```python
from build123d import *

# Parameters (mm, degrees)
F0_W      = 1000
F0_H      = 5.5340008238
F0_H_2    = 212.9319983523
F1_DEPTH  = 25
F2_W      = 900
F2_H      = 124
F3_DEPTH  = 15
F4_W      = 976
F4_H      = 200
F5_DEPTH  = 380
F6_T      = -12
F7_W      = 380
F7_H      = 45
F8_DEPTH  = 5
F9_W      = 380
F9_H      = 45
F10_DEPTH = 5
F11_R     = 4
F12_DEPTH = 12


# Not quite as in the source:
# - a shell that OpenCascade refuses in one call is made with other operations: the cavity is built on its own and cut out


with BuildPart() as f1:
    # F0 (on Front) → F1 (new body)
    with BuildSketch(Plane.XZ):
        with Locations((0, 109.2329995881)):
            Rectangle(F0_W, F0_H)
        Rectangle(F0_W, F0_H_2)
        with Locations((0, -109.2329995881)):
            Rectangle(F0_W, F0_H)
    extrude(amount=F1_DEPTH)

    # F2 (on face) → F3 (cut)
    with BuildSketch(Plane.XZ.offset(25)):
        Rectangle(F2_W, F2_H)
    extrude(amount=-F3_DEPTH, mode=Mode.SUBTRACT)

    # F4 (on face) → F5 (join)
    with BuildSketch(Plane(origin=(0, 0, 0), x_dir=(-1, 0, 0), z_dir=(0, 1, 0))):
        Rectangle(F4_W, F4_H)
    extrude(amount=F5_DEPTH)

    # F6: a shell. OpenCascade refuses it in one call, so the cavity is built on its own and cut out:
    # the body offset inwards by the wall thickness, plus a prism from it out through each open face.
    f6_core = offset(f1.part, amount=F6_T, kind=Kind.INTERSECTION, mode=Mode.PRIVATE)
    f6_exits = [f6_core.faces().sort_by_distance(p)[0] for p in [
        (0, 178, 88),
    ]]
    add(f6_core, mode=Mode.SUBTRACT)
    extrude(f6_exits, amount=-F6_T, mode=Mode.SUBTRACT)

    # F7 (on face) → F8 (join)
    with BuildSketch(Plane(origin=(-488, 0, 0), x_dir=(0, -1, 0), z_dir=(-1, 0, 0))):
        with Locations((-190, 0)):
            Rectangle(F7_W, F7_H)
    extrude(amount=F8_DEPTH)

    # F9 (on face) → F10 (join)
    with BuildSketch(Plane.YZ.offset(488)):
        with Locations((190, 0)):
            Rectangle(F9_W, F9_H)
    extrude(amount=F10_DEPTH)

    # F11 (on face) → F12 (cut, through all)
    with BuildSketch(Plane.XZ.offset(10)):
        with Locations((-55, 0)):
            Circle(F11_R)
        with BuildLine():
            ThreePointArc((59, 0), (55, 4), (51, 0))
            ThreePointArc((51, 0), (55, -4), (59, 0))
        make_face()
    extrude(amount=-F12_DEPTH, mode=Mode.SUBTRACT)


solid = f1.part
```
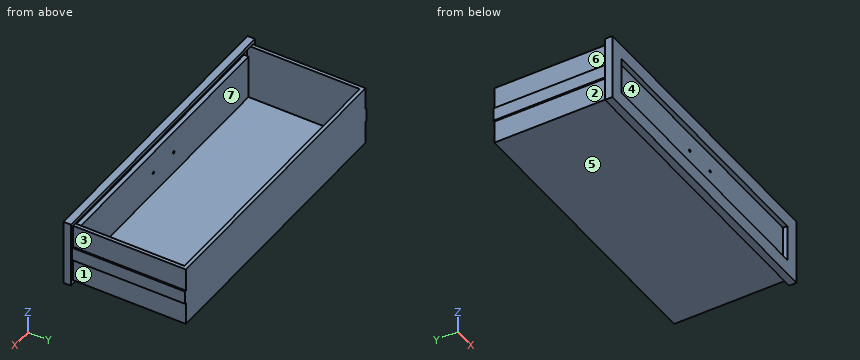
Build history of the part. All positions in model axes, mm. Face numbers are marked on the shaded views. A direction names the side the tool comes from. Give positions to 0.01 mm unless a question says otherwise; leave off trailing zeros. Order: outer loops, then holes, each group sorted by start corner. A loop starts at its lowest first (then second) coordinate and runs counter-clockwise, first axis right, second up. Notation, with made-up numbers: M 34,34 L 73,34 A15 ccw 73,47 Z; hole C 37.25,15.5 d4. An arc over 180 degrees is marked long. Return JSON: item names as keys, results as strings.
Q1. Band-saw the part on C-C (x = 178.5). Give the cut face in (y, z).
Answer list:
{"outline": "M -25,-112 L 0,-112 L 0,-100 L 380,-100 L 380,100 L 368,100 L 368,-88 L -12,-88 L -12,-100 L -13,-100 L -13,-74 L 2,-74 L 2,74 L -13,74 L -13,100 L 0,100 L 0,112 L -25,112 L -25,62 L -10,62 L -10,-62 L -25,-62 Z"}
Q2. 3-axis set-ups, long thin cutter, end or side, ignore diameter. For the marked faces 1, 2, 3 and 4: which of +Z, -Z, +X, -X, +Y, -Y reach the whole face in a straight line?
Answer list:
{"face 1": "-Z, +X, +Y", "face 2": "-Z, -X, +Y", "face 3": "+Z, +X, +Y", "face 4": "-Y"}
Q3. Flat gauge pins, fed straight in: pin 1 (2 mm diameter, centred on x = -4, y = 129, fed in from +Z); pin 2 (10 mm diameter, centred on y = 283, z = 61, fed in from -X); pin 3 (5 mm diameter, centred on y = 191.5, z = 17.5, fed in from -X). Where does each tip first touch, or does it go through?
Answer list:
{"pin 1": "stops at z = -88", "pin 2": "stops at x = -488", "pin 3": "stops at x = -493"}
Q4. Wall check: probe 1 along Z at (x, y) = (-55, -6); probe 2 along X at (y, z) = (-5.5, 52.5); probe 3 along X at (y, z) = (334.5, -53). Give the ranges that are in metal, low to high. Write a range as from..to.
Answer list:
{"probe 1": "z = -112..-88, -74..-4, 4..74, 100..112", "probe 2": "x = -500..-476, -462..462, 476..500", "probe 3": "x = -488..-476, 476..488"}
Q5. Two-plate mould, pull along X, no slides. Class the marked faces 5, 6 and 7: pulls with the +X half, pulls with the -X half, needs draft (parallel to the pull), parting line crosses it, or undercut.
Answer list:
{"face 5": "needs draft", "face 6": "pulls with the -X half", "face 7": "undercut"}
Q6. Band-saw the part on B-B (y = 35). Give the cut face in (x, z).
Answer list:
{"outline": "M -493,-22.5 L -488,-22.5 L -488,-100 L 488,-100 L 488,-22.5 L 493,-22.5 L 493,22.5 L 488,22.5 L 488,100 L 476,100 L 476,-88 L -476,-88 L -476,100 L -488,100 L -488,22.5 L -493,22.5 Z"}
Q7. Band-saw the part on A-A (z = -43). Give the cut face in (x, y), then the cut area to 3 significant figures.
Answer list:
{"outline": "M -500,-25 L -450,-25 L -450,-10 L 450,-10 L 450,-25 L 500,-25 L 500,0 L 488,0 L 488,380 L -488,380 L -488,0 L -500,0 Z; hole M -488,-13 L -462,-13 L -462,2 L 462,2 L 462,-13 L 488,-13 L 488,-12 L 476,-12 L 476,368 L -476,368 L -476,-12 L -488,-12 Z", "area": "33,500 mm^2"}
